Geometry: final body of the model. Coordinates: model frame, mm. Give positions to 0.01 mm unless a question says otherwise; leave off trailing zeros. Write each loop counter-clockwise with the first axis right and the second up, starting at its lowest first coordinate (ties: lowest second). Pieces come first, ordered by that corner, then holes. Notation, with made-up numbers: (-24.5, 50) -> (-10.5, 50) arc R11 ccw to (-10.5, 60) -> close; hole circle Ø11 at (30.5, 51.5). An arc over 180 degrees is marked (long way). Answer in a Markdown table with one row per item. Add a question column.
Item 1: Section query D-D on y = 60. Output: boundary loops of the cut face in (x, z), plus the area to 3 significant figures.
Item 2: Section query C-C on z = 3.5. Output: boundary loops of the cut face in (x, y) (1 decimal).
Item 3: Section query B-B on x = 10.16. Output: boundary loops of the cut face in (y, z).
Item 4: Draft query along Y for faces 1 (the flat face through (56, 49, 0)), 2 (the cylindrical face through (105.832, 9.731, 3.219)), 3 (the flat face through (58, 95.91, 3)). Return one class per face: +Y half, -Y half, draft (parallel to the pull), parting line (faces both ways), or undercut.
Item 5: Material intervals for probe 1 along X at (y, z) = (10.16, 2.25); probe 2 along X at (y, z) = (72, 1); probe 3 along X at (y, z) = (62.5, 2.5), sorted ascending. Write a range as from..to.
Item 6: Section query A-A on y = 10.16. Output: boundary loops of the cut face in (x, z).
Autodesk Inventor part; units mm, degrees
ref_plane "Work Plane1" through (0, 0, -6.35) normal (0, 0, 1) x (1, 0, 0)
ref_plane "Work Plane2" through (0, 0, -41.875) normal (0, 0, 1) x (1, 0, 0)
ref_plane "Work Plane3" through (0, 0, -35.525) normal (0, 0, 1) x (1, 0, 0)
sketch "Sketch1" plane through (0, 0, 0) normal (0, 0, 1) x (1, 0, 0)
  line L0 (0, 0) -> (114.0582, 0)
  line L1 (114.0582, 0) -> (114.0582, 95.9104)
  line L2 (114.0582, 95.9104) -> (0, 95.9104)
  line L3 (0, 95.9104) -> (0, 0)
  line L4 (59.1, 17.1) -> (59.1, 59.1) construction
  line L5 (59.1, 59.1) -> (17.1, 59.1) construction
  line L6 (17.1, 59.1) -> (17.1, 17.1) construction
  line L7 (17.1, 17.1) -> (59.1, 17.1) construction
  line L8 (59.1, 17.1) -> (17.1, 59.1) construction
  line L9 (59.1, 59.1) -> (17.1, 17.1) construction
  circle A0 centre (38.1, 38.1) radius 38.1 construction
  circle A1 centre (38.1, 38.1) radius 20.2 construction
  line L10 (45.4323, 38.1) -> (41.7662, 31.75) construction
  line L11 (41.7662, 31.75) -> (34.4338, 31.75) construction
  line L12 (34.4338, 31.75) -> (30.7677, 38.1) construction
  line L13 (30.7677, 38.1) -> (34.4338, 44.45) construction
  line L14 (34.4338, 44.45) -> (41.7662, 44.45) construction
  line L15 (41.7662, 44.45) -> (45.4323, 38.1) construction
  circle A2 centre (38.1, 38.1) radius 21.59 construction
  line L16 (38.1, 38.1) -> (81.0382, 62.8904) construction
  circle A3 centre (81.0382, 62.8904) radius 27.94 construction
  circle A4 centre (81.0382, 62.8904) radius 23.8125 construction
  circle A5 centre (81.0382, 62.8904) radius 17.4625
  circle A6 centre (38.1, 38.1) radius 14.2875 construction
  line L17 (85.0105, 18.6054) -> (38.1, 38.1) construction
  circle A7 centre (81.0382, 62.8904) radius 33.02 construction
  circle A8 centre (38.1, 38.1) radius 25.4 construction
  circle A9 centre (38.1, 38.1) radius 9.525 construction
  line L18 (81.0382, 62.8904) -> (81.0382, 42.1545) construction
  circle A10 centre (81.0382, 42.1545) radius 2.0828 construction
  circle A11 centre (39.5622, 74.901) radius 10.16 construction
  circle A12 centre (39.5622, 74.901) radius 6.35 construction
  circle A13 centre (81.0382, 42.1545) radius 6.35 construction
  circle A14 centre (38.1, 38.1) radius 26.67 construction
  line L19 (85.0105, 18.6054) -> (87.4474, 24.4692) construction
  line L20 (85.0105, 18.6054) -> (82.5737, 12.7416) construction
  line L21 (87.4474, 24.4692) -> (77.6267, 28.5504) construction
  line L22 (82.5737, 12.7416) -> (72.2567, 17.029) construction
  circle A15 centre (103.8982, 10.16) radius 10.16 construction
  circle A16 centre (103.8982, 10.16) radius 6.35 construction
  circle A17 centre (10.16, 10.16) radius 10.16 construction
  circle A18 centre (38.1, 38.1) radius 32.258 construction
  circle A19 centre (10.16, 10.16) radius 6.35 construction
  point P0 (20.1395, 56.0605)
  point P1 (56.0605, 20.1395)
  point P2 (81.0382, 44.2373)
  point P3 (81.0382, 45.4279)
  point P4 (98.9961, 73.2584)
  point P5 (63.0804, 73.2584)
  point P6 (81.0382, 48.5045)
  point P7 (79.1467, 21.0422)
  dimension "d10" = 34.925
  dimension "d17" = 4.1656
  dimension "d25" = 12.7
  dimension "d0" = 42
  dimension "d1" = 42
  dimension "d2" = 76.2
  dimension "d3" = 40.4
  dimension "d4" = 12.7
  dimension "d5" = 43.18
  dimension "d6" = 55.88
  dimension "d7" = 49.5808
  dimension "d8" = 47.625
  dimension "d11" = 28.575
  dimension "d13" = 30
  dimension "d14" = 5.08
  dimension "d15" = 50.8
  dimension "d16" = 19.05
  dimension "d18" = 1.1906
  dimension "d21" = 360
  dimension "d23" = 20.32
  dimension "d24" = 12.7
  dimension "d26" = 3.0766
  dimension "d30" = 5.08
  dimension "d33" = 50.8
  dimension "d34" = 6.35
  dimension "d35" = 6.35
  dimension "d36" = 20.32
  dimension "d37" = 64.516
  dimension "d38" = 12.7
ref_plane "Work Plane1" through (0, 0, -6.35) normal (0, 0, 1) x (1, 0, 0)
ref_plane "Work Plane2" through (0, 0, -41.875) normal (0, 0, 1) x (1, 0, 0)
ref_plane "Work Plane3" through (0, 0, -35.525) normal (0, 0, 1) x (1, 0, 0)
ref_plane "Work Plane4" through (0, 0, -92.675) normal (0, 0, 1) x (1, 0, 0)
ref_plane "Work Plane5" through (0, 0, -99.025) normal (0, 0, 1) x (1, 0, 0)
sketch "Sketch2" plane through (0, 0, -6.35) normal (0, 0, 1) x (1, 0, 0)
  line L0 (114.0582, 95.9104) -> (0, 95.9104)
  line L1 (0, 95.9104) -> (0, 0)
  line L2 (0, 0) -> (114.0582, 0)
  line L3 (114.0582, 0) -> (114.0582, 95.9104)
  circle A0 centre (81.0382, 62.8904) radius 17.4625
  circle A1 centre (38.1, 38.1) radius 9.525
sketch "Sketch3" plane through (0, 0, -41.875) normal (0, 0, 1) x (1, 0, 0)
  line L0 (114.0582, 95.9104) -> (0, 95.9104)
  line L1 (114.0582, 0) -> (114.0582, 95.9104)
  circle A0 centre (81.0382, 62.8904) radius 17.4625
  line L2 (0, 0) -> (114.0582, 0)
  line L3 (0, 95.9104) -> (0, 0)
  circle A1 centre (38.1, 38.1) radius 14.2875
sketch "Sketch4" plane through (0, 0, -35.525) normal (0, 0, 1) x (1, 0, 0)
  line L0 (114.0582, 95.9104) -> (0, 95.9104)
  line L1 (0, 95.9104) -> (0, 0)
  line L2 (0, 0) -> (114.0582, 0)
  line L3 (114.0582, 0) -> (114.0582, 95.9104)
  circle A0 centre (81.0382, 62.8904) radius 17.4625
  circle A1 centre (38.1, 38.1) radius 14.2875
sketch "Sketch5" plane through (0, 0, -92.675) normal (0, 0, 1) x (1, 0, 0)
  line L0 (0, 95.9104) -> (0, 0)
  line L1 (114.0582, 95.9104) -> (0, 95.9104)
  line L2 (0, 0) -> (114.0582, 0)
  line L3 (114.0582, 0) -> (114.0582, 95.9104)
  circle A0 centre (81.0382, 62.8904) radius 17.4625
sketch "Sketch6" plane through (0, 0, -99.025) normal (0, 0, 1) x (1, 0, 0)
  line L0 (0, 95.9104) -> (0, 0)
  line L1 (0, 0) -> (114.0582, 0)
  line L2 (114.0582, 0) -> (114.0582, 95.9104)
  line L3 (114.0582, 95.9104) -> (0, 95.9104)
  circle A0 centre (81.0382, 62.8904) radius 17.4625
extrude "Extrusion1" add sketch "Sketch1" along normal blind 6.35
hole "Hole1" at (81.0382, 42.1545, 0) at (98.9961, 73.2584, 0) at (63.0804, 73.2584, 0) direction (0, 0, 1) diameter 3.9624 end through all
hole "Hole2" at (39.5622, 74.901, 0) at (10.16, 10.16, 0) at (103.8982, 10.16, 0) direction (0, 0, 1) diameter 3.9624 end through all
equation "\"d30\" = d14"
properties part number "Main Outline"
Findings below:
| question | item | result |
|---|---|---|
| 1 | outline | (0, 0) -> (63.82, 0) -> (63.82, 6.35) -> (0, 6.35) -> close; (98.26, 0) -> (114.06, 0) -> (114.06, 6.35) -> (98.26, 6.35) -> close |
| 1 | area | 506 mm^2 |
| 2 | outline | (0, 0) -> (114.1, 0) -> (114.1, 95.9) -> (0, 95.9) -> close; hole circle Ø4 at (10.2, 10.2); hole circle Ø4 at (39.6, 74.9); hole circle Ø4 at (63.1, 73.3); hole circle Ø34.9 at (81, 62.9); hole circle Ø4 at (81, 42.2); hole circle Ø4 at (99, 73.3); hole circle Ø4 at (103.9, 10.2) |
| 3 | outline | (0, 0) -> (8.18, 0) -> (8.18, 6.35) -> (0, 6.35) -> close; (12.14, 0) -> (95.91, 0) -> (95.91, 6.35) -> (12.14, 6.35) -> close |
| 4 | face 1 | draft |
| 4 | face 2 | undercut |
| 4 | face 3 | +Y half |
| 5 | probe 1 | x = 0..8.18, 12.14..101.92, 105.88..114.06 |
| 5 | probe 2 | x = 0..61.55, 64.61..66.14, 95.94..97.47, 100.53..114.06 |
| 5 | probe 3 | x = 0..63.58, 98.5..114.06 |
| 6 | outline | (0, 0) -> (8.18, 0) -> (8.18, 6.35) -> (0, 6.35) -> close; (12.14, 0) -> (101.92, 0) -> (101.92, 6.35) -> (12.14, 6.35) -> close; (105.88, 0) -> (114.06, 0) -> (114.06, 6.35) -> (105.88, 6.35) -> close |
